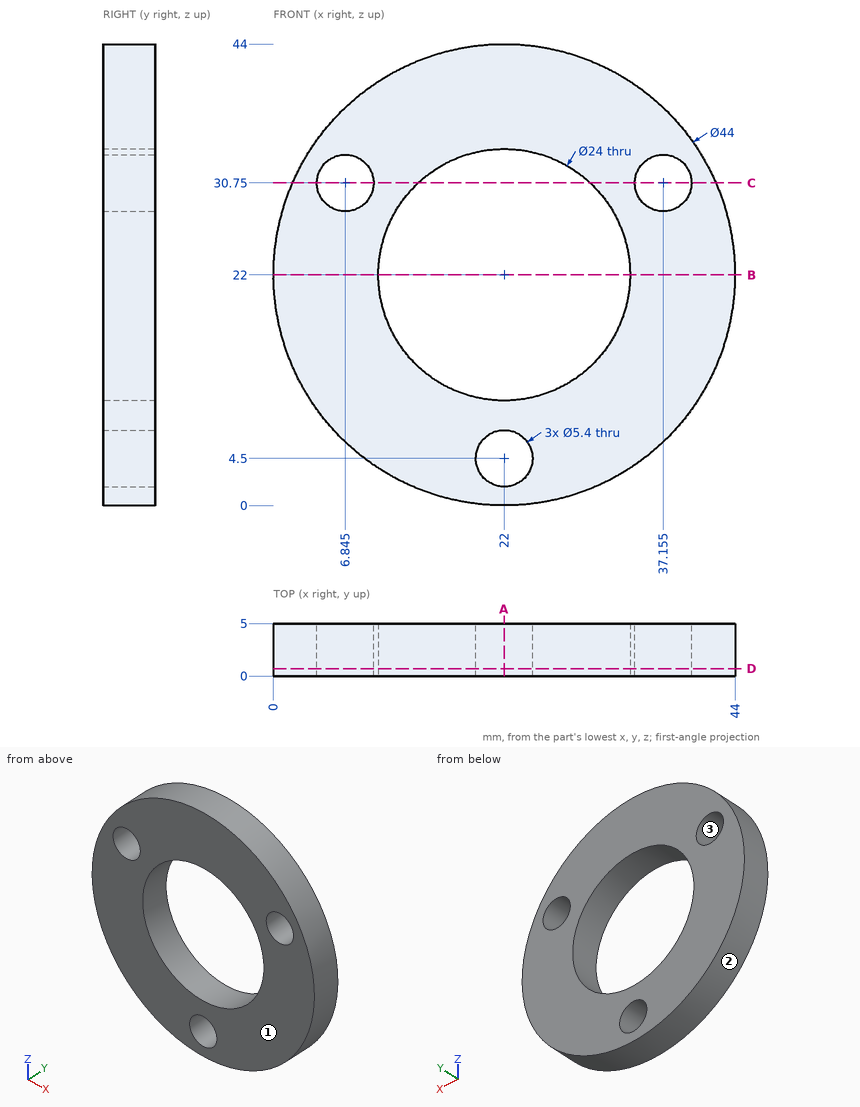
Answer from the drawing. Dimensions are ordinates in mm from the lowest x, y and z of the part. Give positions to 0.01 mm unless a question says otherwise; leave off trailing zeros. Write each loop counter-clockwise with the first axis right and the second up, starting at its lowest first coordinate (ties: lowest second). Pieces come first, ordered by that corner, then holes. Notation, with made-up numbers: (65, 64) - (92, 64) arc R29 cw to (92, 98) - close; hole circle Ø6 at (72.25, 40). An arc over 180 degrees is marked (long way). One line per item, written item: value. Start each with the question number.
1. Find section C-C (z = 30.75). Write down the section's boundary in (x, y) (1 decimal).
2. For a pull along Z with two mould halves and no side action, classify the marked faces 1, 2 and 3 as +Z half, -Z half, draft (parallel to the pull), parting line (faces both ways), or undercut.
3. Given pin 1 (2 mm diameter, centred on y = 4.5, z = 6.5, fed in from -X) (1 decimal), flat-ended and moving along its own axis, determine where the tip first touches the part or whether it passes through.
4. Find section D-D (y = 0.7). State how many separate pieces and enclosed holes the cut face has.
5. Find section A-A (x = 22). Write down the section's boundary in (y, z).
6. Find section B-B (z = 22). Write down the section's boundary in (x, y).
7. Consider probe 1 along X at (y, z) = (2.9, 30.75) (1 decimal); probe 2 along X at (y, z) = (4.05, 22); probe 3 along Z at (x, y) = (14.5, 3.15). Determine where each line is inside the solid, lowest interval first.
Geometry results:
1. outline: (1.8, 0) - (4.1, 0) - (4.1, 5) - (1.8, 5) - close; (9.5, 0) - (13.8, 0) - (13.8, 5) - (9.5, 5) - close; (30.2, 0) - (34.5, 0) - (34.5, 5) - (30.2, 5) - close; (39.9, 0) - (42.2, 0) - (42.2, 5) - (39.9, 5) - close
2. face 1: draft
2. face 2: parting line
2. face 3: undercut
3. pin 1: x = 5.5
4. separate pieces: 1
4. enclosed holes: 4
5. outline: (0, 0) - (5, 0) - (5, 1.8) - (0, 1.8) - close; (0, 7.2) - (5, 7.2) - (5, 10) - (0, 10) - close; (0, 34) - (5, 34) - (5, 44) - (0, 44) - close
6. outline: (0, 0) - (10, 0) - (10, 5) - (0, 5) - close; (34, 0) - (44, 0) - (44, 5) - (34, 5) - close
7. probe 1: 1.8 to 4.1, 9.5 to 13.8, 30.2 to 34.5, 39.9 to 42.2
7. probe 2: 0 to 10, 34 to 44
7. probe 3: 1.32 to 12.63, 31.37 to 42.68
